```python
from build123d import *

# Parameters (mm, degrees)
SKETCH1_W           = 30
SKETCH1_H           = 30
BOSS_EXTRUDE1_DEPTH = 5
CUT_EXTRUDE1_REACH  = 23.794
SKETCH2_R           = 1
FILLET1_R           = 3
SKETCH3_R           = 12.5
BOSS_EXTRUDE2_DEPTH = 5.5
SKETCH4_R           = 12.5
SKETCH4_R_2         = 10.5
BOSS_EXTRUDE3_DEPTH = 5
CUT_EXTRUDE2_REACH  = 25.67
SKETCH5_R           = 6


with BuildPart() as part:
    # Sketch1 → Boss-Extrude1 (new body)
    with BuildSketch(Plane(origin=(0, 0, 0), x_dir=(1, 0, 0), z_dir=(0, 1, 0))):
        Rectangle(SKETCH1_W, SKETCH1_H)
    extrude(amount=BOSS_EXTRUDE1_DEPTH)

    # Sketch2 → Cut-Extrude1 (cut, up to next)
    with BuildSketch(Plane(origin=(0, 5, 0), x_dir=(1, 0, 0), z_dir=(0, 1, 0)), mode=Mode.PRIVATE) as cut_extrude1_sk1:
        with Locations(Location((-12, 12, 0), (0, 0, 270))):
            Circle(SKETCH2_R)
    cut_extrude1_tool1 = extrude(cut_extrude1_sk1.sketch, amount=-CUT_EXTRUDE1_REACH, mode=Mode.PRIVATE) & part.part
    # Sketch2 → Cut-Extrude1 (cut, up to next)
    with BuildSketch(Plane(origin=(0, 5, 0), x_dir=(1, 0, 0), z_dir=(0, 1, 0)), mode=Mode.PRIVATE) as cut_extrude1_sk2:
        with Locations(Location((12, 12, 0), (0, 0, 270))):
            Circle(SKETCH2_R)
    cut_extrude1_tool2 = extrude(cut_extrude1_sk2.sketch, amount=-CUT_EXTRUDE1_REACH, mode=Mode.PRIVATE) & part.part
    # Sketch2 → Cut-Extrude1 (cut, up to next)
    with BuildSketch(Plane(origin=(0, 5, 0), x_dir=(1, 0, 0), z_dir=(0, 1, 0)), mode=Mode.PRIVATE) as cut_extrude1_sk3:
        with Locations(Location((-12, -12, 0), (0, 0, 270))):
            Circle(SKETCH2_R)
    cut_extrude1_tool3 = extrude(cut_extrude1_sk3.sketch, amount=-CUT_EXTRUDE1_REACH, mode=Mode.PRIVATE) & part.part
    # Sketch2 → Cut-Extrude1 (cut, up to next)
    with BuildSketch(Plane(origin=(0, 5, 0), x_dir=(1, 0, 0), z_dir=(0, 1, 0)), mode=Mode.PRIVATE) as cut_extrude1_sk4:
        with Locations(Location((12, -12, 0), (0, 0, 270))):
            Circle(SKETCH2_R)
    cut_extrude1_tool4 = extrude(cut_extrude1_sk4.sketch, amount=-CUT_EXTRUDE1_REACH, mode=Mode.PRIVATE) & part.part
    add(cut_extrude1_tool1.solids().sort_by_distance((-12, 5, -12))[0], mode=Mode.SUBTRACT)
    add(cut_extrude1_tool2.solids().sort_by_distance((12, 5, -12))[0], mode=Mode.SUBTRACT)
    add(cut_extrude1_tool3.solids().sort_by_distance((-12, 5, 12))[0], mode=Mode.SUBTRACT)
    add(cut_extrude1_tool4.solids().sort_by_distance((12, 5, 12))[0], mode=Mode.SUBTRACT)

    # Fillet1
    fillet1_edges = [part.edges().sort_by_distance(p)[0] for p in [
        (15, 2.5, 15),
        (-15, 2.5, 15),
        (-15, 2.5, -15),
        (15, 2.5, -15),
    ]]
    fillet(fillet1_edges, radius=FILLET1_R)

    # Sketch3 → Boss-Extrude2 (add)
    with BuildSketch(Plane(origin=(0, 5, 0), x_dir=(1, 0, 0), z_dir=(0, 1, 0))):
        with Locations(Location((0, 0, 0), (0, 0, 90))):
            Circle(SKETCH3_R)
    extrude(amount=BOSS_EXTRUDE2_DEPTH)

    # Sketch4 → Boss-Extrude3 (add)
    with BuildSketch(Plane(origin=(0, 10.5, 0), x_dir=(1, 0, 0), z_dir=(0, 1, 0))):
        with Locations(Location((0, 0, 0), (0, 0, 90))):
            Circle(SKETCH4_R)
        with Locations(Location((0, 0, 0), (0, 0, 270))):
            Circle(SKETCH4_R_2, mode=Mode.SUBTRACT)
    extrude(amount=BOSS_EXTRUDE3_DEPTH)

    # Sketch5 → Cut-Extrude2 (cut, up to next)
    with BuildSketch(Plane(origin=(0, 10.5, 0), x_dir=(1, 0, 0), z_dir=(0, 1, 0)), mode=Mode.PRIVATE) as cut_extrude2_sk1:
        with Locations(Location((0, 0, 0), (0, 0, 270))):
            Circle(SKETCH5_R)
    cut_extrude2_tool1 = extrude(cut_extrude2_sk1.sketch, amount=-CUT_EXTRUDE2_REACH, mode=Mode.PRIVATE) & part.part
    add(cut_extrude2_tool1.solids().sort_by_distance((0, 10.5, 0))[0], mode=Mode.SUBTRACT)


solid = part.part
```
Build history of the part. All positions in model axes, mm. A direction names the side the tool comes from. Give positions to 0.01 mm unless a question says otherwise; leave off trailing zeros. Loops run counter-clockwise (first coordinate to the right, second up) from the corner with the lowest first, then second, coordinate; pieces in that order, holes last. Notation, with made-up numbers: (7.5, 53) -> (56.5, 53) arc R11 ccw to (56.5, 60) -> close; hole circle Ø6 at (16.5, 81). An arc over 180 degrees is marked (long way). One line per question, with ' | ' between items. Start each with the question number.
1) Probe L1, parallel to X at y = 1.95, z = -12; L2, parallel to Y at x = 6.5, z = 0.5; L3, parallel to Y at x = 11.25, z = -7.5. List the from-to ranges inside material, lowest first.
2) Cut at B-B (z = -4). Give the cut face in (x, y).
3) Pin check, flat tips, straight feed: pin 1 (3 mm diameter, centred on x = -12, z = -12, fed in from +Y); pin 2 (6.5 mm diameter, centred on x = -3, z = 2, fed in from +Y); pin 3 (6 mm diameter, centred on y = 9.5, z = 10.5, fed in from +X). Stop position of each tip, or through.
4) Cut at A-A (x = 0). Give the cut face in (y, z).
5) Cut at C-C (x = 11.5). Give the cut face in (y, z).
6) 3-axis set-ups, long thin cutter, end or side, ignore diameter. For faces 1 (the cylindrical face through (-3.755, 10.176, -11.923)), 2 (the flat face through (0, 2, -15)): which of +Z, -Z, +X, -X, +Y, -Y reach the whole face in a straight line?
7) Cut at D-D (y = 12.5). Give the cut face in (x, z), plus the area to 3 significant figures.
8) Two-plate mould, pull along X, no slides. Class faces 3 (the flat face through (-14, 5, 0)), 4 (the cylindrical face through (11.4, 2.5, -12.8)), 5 (the cylindrical face through (14.1, 2.54, -14.14)): released by +X, released by -X, zero draft, split by the parting line, or undercut.
Return value:
1) L1: -15 to -13, -11 to 11, 13 to 15 | L2: 0 to 10.5 | L3: 0 to 5
2) outline: (-15, 0) -> (-4.47, 0) -> (-4.47, 10.5) -> (-9.71, 10.5) -> (-9.71, 15.5) -> (-11.84, 15.5) -> (-11.84, 5) -> (-15, 5) -> close; (4.47, 0) -> (15, 0) -> (15, 5) -> (11.84, 5) -> (11.84, 15.5) -> (9.71, 15.5) -> (9.71, 10.5) -> (4.47, 10.5) -> close
3) pin 1: y = 5 | pin 2: y = 10.5 | pin 3: x = 10
4) outline: (0, -15) -> (5, -15) -> (5, -12.5) -> (15.5, -12.5) -> (15.5, -10.5) -> (10.5, -10.5) -> (10.5, -6) -> (0, -6) -> close; (0, 6) -> (10.5, 6) -> (10.5, 10.5) -> (15.5, 10.5) -> (15.5, 12.5) -> (5, 12.5) -> (5, 15) -> (0, 15) -> close
5) outline: (0, -15) -> (5, -15) -> (5, -12.87) -> (0, -12.87) -> close; (0, -11.13) -> (5, -11.13) -> (5, -4.9) -> (15.5, -4.9) -> (15.5, 4.9) -> (5, 4.9) -> (5, 11.13) -> (0, 11.13) -> close; (0, 12.87) -> (5, 12.87) -> (5, 15) -> (0, 15) -> close
6) face 1: +Y | face 2: -Z, +X, -X, +Y, -Y
7) outline: circle Ø25 at (0, 0); hole circle Ø21 at (0, 0) | area: 145 mm^2
8) face 3: zero draft | face 4: undercut | face 5: released by +X
